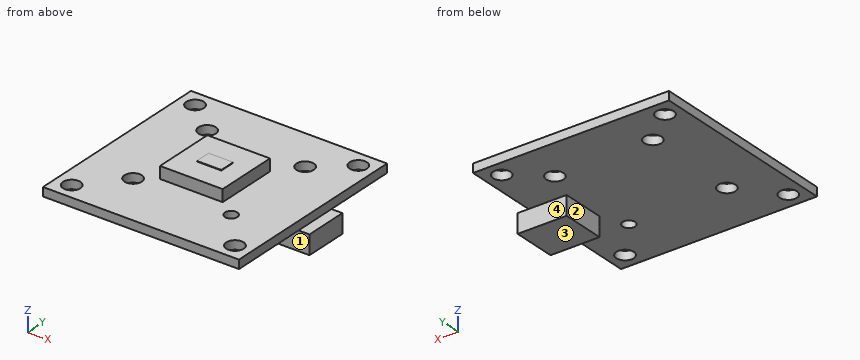
Autodesk Inventor part; units mm, degrees
ref_plane "YZ Plane" through (0, 0, 0) normal (1, 0, 0) x (0, 1, 0)
ref_plane "XZ Plane" through (0, 0, 0) normal (0, 1, 0) x (-1, 0, 0)
ref_plane "XY Plane" through (0, 0, 0) normal (0, 0, 1) x (1, 0, 0)
sketch "Sketch1" plane through (0, 0, 0) normal (0, 0, 1) x (1, 0, 0)
  line L0 (-25.2, 0) -> (25.2, 0) construction
  line L1 (0, -25.2) -> (0, 25.2) construction
  line L2 (-18, 18) -> (18, 18)
  line L3 (18, 18) -> (18, -18)
  line L4 (18, -18) -> (-18, -18)
  line L5 (-18, -18) -> (-18, 18)
  point P0 (0, 0)
  point P1 (0, 18)
  point P2 (18, 0)
  dimension "d0" = 36
  dimension "d1" = 36
extrude "Extrusion1" add sketch "Sketch1" along normal blind 1.6
sketch "Sketch2" plane through (0, 0, 1.6) normal (0, 0, 1) x (1, 0, 0)
  point P0 (0, 0)
  point P1 (-15, 15)
  dimension "d4" = 15
  dimension "d5" = 15
hole "Hole1" at (-15, 15, 1.6) direction (0, 0, -1) diameter 3.2 end through all
pattern_circular "Circular Pattern1" count 4 over 360 about axis through (0, 0, -10) along (0, 0, 1) of "Hole1"
sketch "Sketch3" plane through (0, 0, 1.6) normal (0, 0, 1) x (1, 0, 0)
  line L0 (-25.2, 0) -> (25.2, 0) construction
  line L1 (0, -25.2) -> (0, 25.2) construction
  line L2 (-2.256, 1.44) -> (2.256, 1.44)
  line L3 (2.256, 1.44) -> (2.256, -1.44)
  line L4 (2.256, -1.44) -> (-2.256, -1.44)
  line L5 (-2.256, -1.44) -> (-2.256, 1.44)
  point P0 (0, 0)
  point P1 (0, 1.44)
  point P2 (2.256, 0)
  dimension "d16" = 4.512
  dimension "d17" = 2.88
extrude "Extrusion2" add sketch "Sketch3" along normal blind 2.3
sketch "Sketch4" plane through (0, 0, 1.6) normal (0, 0, 1) x (1, 0, 0)
  line L0 (-5.75, 5.75) -> (5.75, 5.75)
  line L1 (5.75, 5.75) -> (5.75, -5.75)
  line L2 (5.75, -5.75) -> (-5.75, -5.75)
  line L3 (-5.75, -5.75) -> (-5.75, 5.75)
  line L4 (-25.2, 0) -> (25.2, 0) construction
  line L5 (0, -25.2) -> (0, 25.2) construction
  point P0 (0, 0)
  point P1 (0, 5.75)
  point P2 (5.75, 0)
  dimension "d20" = 11.5
  dimension "d21" = 11.5
extrude "Extrusion3" add sketch "Sketch4" along normal blind 2.2
sketch "Sketch5" plane through (0, 0, 1.6) normal (0, 0, 1) x (1, 0, 0)
  point P0 (0, 0)
sketch "Sketch6" plane through (0, 0, 0) normal (0, 0, -1) x (-1, 0, 0)
  line L0 (25.2, 0) -> (-25.2, 0)
  line L1 (0, -25.2) -> (0, 25.2)
  line L2 (-20, 4.5) -> (-11, 4.5)
  line L3 (-11, 4.5) -> (-11, -3.5)
  line L4 (-11, -3.5) -> (-20, -3.5)
  line L5 (-20, -3.5) -> (-20, 4.5)
  line L6 (-18, 18) -> (-18, -18)
  line L7 (-18, -18) -> (18, -18)
  point P0 (0, 0)
  point P1 (-11, 0.5)
  dimension "d24" = 9
  dimension "d25" = 8
  dimension "d26" = 2
  dimension "d58" = 18.5
extrude "Extrusion4" add sketch "Sketch6" along normal blind 3.5 contours L3 L4 L6 L0 | L0 L6 L2 L3 | L6 L4 L5 L0 | L0 L5 L2 L6
sketch "Sketch7" plane through (0, 0, 1.6) normal (0, 0, 1) x (1, 0, 0)
  line L0 (-25.6, 0) -> (27.6, 0)
  line L1 (0, -25.2) -> (0, 25.2)
  line L2 (18, -18) -> (18, 18)
  line L3 (18, -18) -> (-18, -18)
  circle A0 centre (9, -8) radius 1.15
  circle A1 centre (-9, -8) radius 1.6
  circle A2 centre (-9, 10) radius 1.6
  circle A3 centre (9, 10) radius 1.6
  line L4 (-18, 18) -> (18, 18)
  point P0 (0, 0)
  dimension "d44" = 3.2
  dimension "d45" = 3.2
  dimension "d46" = 3.2
  dimension "d47" = 2.3
  dimension "d48" = 10
  dimension "d49" = 10
  dimension "d50" = 9
  dimension "d51" = 9
  dimension "d52" = 8
  dimension "d53" = 8
  dimension "d54" = 18
  dimension "d55" = 18
extrude "Extrusion5" cut sketch "Sketch7" against normal through all contours A0 | A1 | A2 | A3
equation "\"d20\" = d21"
properties part number "F103" material "Acetal Resin, Black"
Design review of the part built by this model. Coordinates are the model's own, in mm. Face numbers are marked on the shaded views. A direction names the side the tool comes from. Give positions to 0.01 mm unless a question says otherwise; leave off trailing zeros. Order: outer loops, then holes, each group sorted by start corner. A loop starts at its lowest first (then second) coordinate and runs counter-clockwise, first axis right, second up. Notation, with made-up numbers: (-30.75, 23.25) - (-26.75, 23.25) arc R9 cw to (-26.75, 31.25) - close; hole circle Ø4 at (57, 28.5). An arc over 180 degrees is marked (long way). Use a Markdown table: item, result. Add a question column.
(1) Add section A-A on x = 9. Give the boundary of the cut face in (y, z).
(2) Machinability: for the marked faces 1, 2, 3 and 4, which of the approach directions +Z, -Z, +X, -X, +Y, -Y give a long, thin tool a straight path to every point of the face, cutting with its end or side? Answer none if there is none.
(3) Add section B-B on y = 15. Give the boundary of the cut face in (x, z).
(4) Wall thickness on probe 1 along Y at (x, z) = (9, 0.3); probe 2 along X at (y, z) = (-15, 0.5); probe 3 along Y at (x, z) = (-9, 0.9): over which ranges is each line inside the solid? List them lowest first. Write a range as [from, to].
(5) Add section C-C on x = -5. Give the boundary of the cut face in (y, z), then the cut area to 3 significant figures.
(6) Add section D-D on y = 3. Give the boundary of the cut face in (x, z).
(7) Clearance check with flat-ended pins moving along their axes: P1, Ø5, axis at x = -9, y = -8, coming from the +Z side; P2, Ø11, axis at x = 4, y = 3.5, coming from the -Z side; P3, Ø0.7, axis at x = 2, z = 2.5, coming from the -Y side. State where each tip first meets the part, or that it passes through.
Report:
| question | item | result |
|---|---|---|
| 1 | outline | (-18, 0) - (-9.15, 0) - (-9.15, 1.6) - (-18, 1.6) - close; (-6.85, 0) - (8.4, 0) - (8.4, 1.6) - (-6.85, 1.6) - close; (11.6, 0) - (18, 0) - (18, 1.6) - (11.6, 1.6) - close |
| 2 | face 1 | -Z, +X, -X, -Y |
| 2 | face 2 | -Z, -X, +Y, -Y |
| 2 | face 3 | -Z, +X, -X, +Y, -Y |
| 2 | face 4 | -Z, +X, -X, +Y |
| 3 | outline | (-18, 0) - (-16.6, 0) - (-16.6, 1.6) - (-18, 1.6) - close; (-13.4, 0) - (13.4, 0) - (13.4, 1.6) - (-13.4, 1.6) - close; (16.6, 0) - (18, 0) - (18, 1.6) - (16.6, 1.6) - close |
| 4 | probe 1 | y = [-18, -9.15], [-6.85, 8.4], [11.6, 18] |
| 4 | probe 2 | x = [-18, -16.6], [-13.4, 13.4], [16.6, 18] |
| 4 | probe 3 | y = [-18, -9.6], [-6.4, 8.4], [11.6, 18] |
| 5 | outline | (-18, 0) - (18, 0) - (18, 1.6) - (5.75, 1.6) - (5.75, 3.8) - (-5.75, 3.8) - (-5.75, 1.6) - (-18, 1.6) - close |
| 5 | area | 82.9 mm² |
| 6 | outline | (-18, 0) - (11, 0) - (11, -3.5) - (20, -3.5) - (20, 0) - (18, 0) - (18, 1.6) - (5.75, 1.6) - (5.75, 3.8) - (-5.75, 3.8) - (-5.75, 1.6) - (-18, 1.6) - close |
| 7 | P1 | stops at z = 1.6 |
| 7 | P2 | stops at z = 0 |
| 7 | P3 | stops at y = -5.75 |
